Could you check a few things on this model? Use its own coordinates, in mm. A direction names the side the tool comes from. Round coordinates to 2 decimals unless told otherwise and drop trailing zeros. Loops run counter-clockwise (first coordinate to the right, second up) from the corner with the lowest first, then second, coordinate; pieces in that order, holes last. Notation, with made-up numbers: (1.5, -17.5) - (39.5, -17.5) arc R12 cw to (39.5, -11.5) - close; hole circle Ø4 at (79, 6.25). An arc over 180 degrees is marked (long way). Put each result on its own line as item: value. Start each with the question number.
from build123d import *

# Parameters (mm, degrees)
CHAMFER1_SIZE      = 1
CUT_EXTRUDE1_START = -12
CUT_EXTRUDE1_DEPTH = 12


with BuildPart() as part:
    # Sketch1 → Revolve1 (revolve)
    with BuildSketch(Plane.XY, mode=Mode.PRIVATE) as revolve1_sk:
        Polygon((0, 0), (0, 23), (16, 23), (16, 14), (69, 14), (69, 11), (83, 11), (83, 8), (86, 8), (86, 10), (106, 10), (106, 0), align=None)
    revolve(revolve1_sk.sketch.rotate(Axis((0, 0, 0), (1, 0, 0)), 90), axis=Axis((0, 0, 0), (1, 0, 0)))

    # Chamfer1
    chamfer1_edges = [part.edges().sort_by_distance(p)[0] for p in [
        (106, 0, -10),
    ]]
    chamfer(chamfer1_edges, length=CHAMFER1_SIZE)

    # Sketch2 → Cut-Extrude1 (cut)
    with BuildSketch(Plane.ZY.offset(CUT_EXTRUDE1_START)):
        with BuildLine():
            Line((-15, 17.435595774), (-15, -17.435595774))
            ThreePointArc((-15, -17.435595774), (-23, 0), (-15, 17.435595774))
        make_face()
        with BuildLine():
            Line((15, 17.435595774), (15, -17.435595774))
            ThreePointArc((15, -17.435595774), (23, 0), (15, 17.435595774))
        make_face()
    extrude(amount=CUT_EXTRUDE1_DEPTH, mode=Mode.SUBTRACT)


solid = part.part
Item 1: Suppose I cut it at B-B, the plane y = 0. List the corners of the cut face in (x, z) for me, then the cut area to 3 significant figures.
Item 2: Suppose I cut it at D-D, the plane x = 55. List the corners of the cut face in (y, z) for me, then the cut area to 3 significant figures.
Item 3: Suppose I cut it at A-A, the plane z = 0. List the corners of the cut face in (x, y) for me, then the cut area to 4 significant figures.
Item 4: Thinking about a two-plate mould opening in X: for faces 1 (the face through (84.52, 7.81, -1.73)), 2 (the face through (76.1, 10.74, -2.38)), 3 (the face through (69, 9.3, 6.2)), 4 (the face through (83, 8, -2)), which applies, released by +X, released by -X, zero draft, split by the parting line, or undercut?
Item 5: I need wall thicknesses on line 1 (X direction, y = -10.5, z = -6.5); line 2 (X direction, y = 21.5, z = -0.5); line 3 (Z direction, x = 5.5, y = -17). Which ranges of each line are inside material? Lowest first, please. Write a range as from..to.
Item 6: Will these pins go through, and if not, where does the flat tip stop? P1, Ø3.5, axis at x = 6, y = 3.5, coming from the +Z side; P2, Ø2, axis at y = 10, z = 5, coming from the +X side; P3, Ø1.5, axis at x = 35.5, z = 9.5, coming from the +Y side.
Item 7: On a 3-axis mill with a long thin cutter (end or side, diameter ignored), from which of +Z, -Z, +X, -X, +Y, -Y can I reach the whole of each face in a straight line? I mean faces 5 (the face through (96, 0, -10)), 6 (the face through (6, 0, 15)), 7 (the face through (12, 0, -18)). Say none if no direction works.
Item 8: Suppose I cut it at C-C, the plane x = 97. List the corners of the cut face in (y, z) for me.
Numbers:
1. outline: (0, -15) - (12, -15) - (12, -23) - (16, -23) - (16, -14) - (69, -14) - (69, -11) - (83, -11) - (83, -8) - (86, -8) - (86, -10) - (105, -10) - (106, -9) - (106, 9) - (105, 10) - (86, 10) - (86, 8) - (83, 8) - (83, 11) - (69, 11) - (69, 14) - (16, 14) - (16, 23) - (12, 23) - (12, 15) - (0, 15) - close
1. area: 2,780 mm^2
2. outline: circle Ø28 at (0, 0)
2. area: 616 mm^2
3. outline: (0, -23) - (16, -23) - (16, -14) - (69, -14) - (69, -11) - (83, -11) - (83, -8) - (86, -8) - (86, -10) - (105, -10) - (106, -9) - (106, 9) - (105, 10) - (86, 10) - (86, 8) - (83, 8) - (83, 11) - (69, 11) - (69, 14) - (16, 14) - (16, 23) - (0, 23) - close
3. area: 2,975 mm^2
4. face 1: undercut
4. face 2: zero draft
4. face 3: released by +X
4. face 4: undercut
5. line 1: 0..69
5. line 2: 0..16
5. line 3: -15..15
6. P1: z = 15
6. P2: x = 83
6. P3: y = 10.93
7. face 5: +X
7. face 6: +Z, -X, +Y, -Y
7. face 7: -Z, -X, +Y, -Y
8. outline: circle Ø20 at (0, 0)
